Input: part model. Units: mm. Frame: model coordinates. A direction names the side the tool comes from. Give positions to 0.01 mm unless a question says otherwise; leave off trailing zeros. Loops run counter-clockwise (first coordinate to the right, second up) from the corner with the lowest first, then second, coordinate; pieces in that order, holes last. Notation, with made-up numbers: (-21.75, 16) -> (-7.75, 16) arc R29 cw to (-7.75, 51) -> close; hole circle Ø3 at (-13, -35). An arc over 180 degrees is marked (long way). One line per question, with ' | ' between items.
from build123d import *

# Parameters (mm, degrees)
EXTRUDE_THIN1_DEPTH             = 37.5
EXTRUDE_THIN1_DEPTH_BACK        = 37.5
CUT_EXTRUDE1_REACH              = 44.057
LPATTERN1_COUNT                 = 2
LPATTERN1_PITCH                 = 25
LPATTERN1_COL_COUNT             = 2
LPATTERN1_COL_PITCH             = 25
SCHNITT_LINEAR_START            = -11
SCHNITT_LINEAR_AUSTRAGEN1_DEPTH = 11


with BuildPart() as part:
    # Sketch1 → Extrude-Thin1 (new, two sides: drawn at the far end of the back side and taken through both)
    with BuildSketch(Plane(origin=(0, 0, 0), x_dir=(0, 0, -1), z_dir=(1, 0, 0)).offset(-EXTRUDE_THIN1_DEPTH_BACK)):
        with BuildLine():
            Line((-17.5, 6.5), (-15.5, 6.5))
            ThreePointArc((-15.5, 6.5), (-14.085786438, 5.914213562), (-13.5, 4.5))
            Line((-13.5, 4.5), (-13.5, 2))
            ThreePointArc((-13.5, 2), (-12.914213562, 0.585786438), (-11.5, 0))
            Line((-11.5, 0), (11.5, 0))
            ThreePointArc((11.5, 0), (12.914213562, 0.585786438), (13.5, 2))
            Line((13.5, 2), (13.5, 4.5))
            ThreePointArc((13.5, 4.5), (14.085786438, 5.914213562), (15.5, 6.5))
            Line((15.5, 6.5), (17.5, 6.5))
            Line((17.5, 6.5), (17.5, 7.5))
            Line((17.5, 7.5), (15.5, 7.5))
            ThreePointArc((15.5, 7.5), (13.378679656, 6.621320344), (12.5, 4.5))
            Line((12.5, 4.5), (12.5, 2))
            ThreePointArc((12.5, 2), (12.207106781, 1.292893219), (11.5, 1))
            Line((11.5, 1), (-11.5, 1))
            ThreePointArc((-11.5, 1), (-12.207106781, 1.292893219), (-12.5, 2))
            Line((-12.5, 2), (-12.5, 4.5))
            ThreePointArc((-12.5, 4.5), (-13.378679656, 6.621320344), (-15.5, 7.5))
            Line((-15.5, 7.5), (-17.5, 7.5))
            Line((-17.5, 7.5), (-17.5, 6.5))
        make_face()
    extrude(amount=EXTRUDE_THIN1_DEPTH + EXTRUDE_THIN1_DEPTH_BACK)

    # Sketch2 → Cut-Extrude1 (cut, up to next)
    with BuildSketch(Plane.XZ, mode=Mode.PRIVATE) as cut_extrude1_sk1:
        with BuildLine():
            Line((-5.875, 3.125), (5.875, 3.125))
            ThreePointArc((5.875, 3.125), (9, 0), (5.875, -3.125))
            Line((5.875, -3.125), (-5.875, -3.125))
            ThreePointArc((-5.875, -3.125), (-9, 0), (-5.875, 3.125))
        make_face()
    cut_extrude1_tool1 = extrude(cut_extrude1_sk1.sketch, amount=-CUT_EXTRUDE1_REACH, mode=Mode.PRIVATE) & part.part
    cut_extrude1 = cut_extrude1_tool1.solids().sort_by_distance((0, 0, 0))[0]
    add(cut_extrude1, mode=Mode.SUBTRACT)

    # LPattern1: Cut-Extrude1 ×2
    with Locations(*[(i * LPATTERN1_PITCH, 0, 0) for i in range(1, LPATTERN1_COUNT)]):
        add(cut_extrude1, mode=Mode.SUBTRACT)

    # LPattern1 col: Cut-Extrude1 ×2
    with Locations(*[(-i * LPATTERN1_COL_PITCH, 0, 0) for i in range(1, LPATTERN1_COL_COUNT)]):
        add(cut_extrude1, mode=Mode.SUBTRACT)

    # Skizze1 → Schnitt-Linear austragen1 (cut)
    with BuildSketch(Plane(origin=(37.5, 0, 0), x_dir=(0, 0, -1), z_dir=(1, 0, 0)).offset(SCHNITT_LINEAR_START)):
        with BuildLine():
            Line((-15.5, 7.5), (-17.5, 7.5))
            Line((-17.5, 7.5), (-17.5, 6.5))
            Line((-17.5, 6.5), (-15.5, 6.5))
            ThreePointArc((-15.5, 6.5), (-14.085786438, 5.914213562), (-13.5, 4.5))
            Line((-13.5, 4.5), (-13.5, 2))
            ThreePointArc((-13.5, 2), (-12.914213562, 0.585786438), (-11.5, 0))
            Line((-11.5, 0), (11.5, 0))
            ThreePointArc((11.5, 0), (12.914213562, 0.585786438), (13.5, 2))
            Line((13.5, 2), (13.5, 4.5))
            ThreePointArc((13.5, 4.5), (14.085786438, 5.914213562), (15.5, 6.5))
            Line((15.5, 6.5), (17.5, 6.5))
            Line((17.5, 6.5), (17.5, 7.5))
            Line((17.5, 7.5), (15.5, 7.5))
            ThreePointArc((15.5, 7.5), (13.378679656, 6.621320344), (12.5, 4.5))
            Line((12.5, 4.5), (12.5, 2))
            ThreePointArc((12.5, 2), (12.207106781, 1.292893219), (11.5, 1))
            Line((11.5, 1), (-11.5, 1))
            ThreePointArc((-11.5, 1), (-12.207106781, 1.292893219), (-12.5, 2))
            Line((-12.5, 2), (-12.5, 4.5))
            ThreePointArc((-12.5, 4.5), (-13.378679656, 6.621320344), (-15.5, 7.5))
        make_face()
    extrude(amount=SCHNITT_LINEAR_AUSTRAGEN1_DEPTH, mode=Mode.SUBTRACT)


solid = part.part
1. Section query B-B (z = 0). Output: boundary loops of the cut face in (x, y), then the cut area to 3 significant figures.
Determined:
outline: (-37.5, 0) -> (-34, 0) -> (-34, 1) -> (-37.5, 1) -> close; (-16, 0) -> (-9, 0) -> (-9, 1) -> (-16, 1) -> close; (9, 0) -> (16, 0) -> (16, 1) -> (9, 1) -> close | area: 17.5 mm2
2. Ray query, line 1 along Z through (x, y) = (20.5, 4.25); line 2 along Y through (x, z) = (22, -10.5); line 3 along Z through (x, y) = (-35, 7.25). Return the intervals inside material, ascending. Write a range as from..to.
Determined:
line 1: z = -13.5..-12.5, 12.5..13.5 | line 2: y = 0..1 | line 3: z = -17.5..-14.3, 14.3..17.5
3. Section query A-A (y = 3.5). Output: boundary loops of the cut face in (x, z).
Determined:
outline: (-37.5, -13.5) -> (26.5, -13.5) -> (26.5, -12.5) -> (-37.5, -12.5) -> close; (-37.5, 12.5) -> (26.5, 12.5) -> (26.5, 13.5) -> (-37.5, 13.5) -> close
4. Pull-direction query (Z, two-part tool) for faces 1 (the flat face through (-6, 3, -13.5)), 2 (the flat face through (-6, 6.5, -16)), 3 (the cylindrical face through (-16, 0.5, 0.1)); classes: pulls with the +Z half, pulls with the -Z half, needs draft (parallel to the pull), parting line crosses it, or undercut.
Determined:
face 1: pulls with the -Z half | face 2: needs draft | face 3: undercut
5. Section query C-C (x = -33). Output: boundary loops of the cut face in (y, z), then the cut area to 3 significant figures.
Determined:
outline: (0, -11.5) arc R2 ccw to (2, -13.5) -> (4.5, -13.5) arc R2 cw to (6.5, -15.5) -> (6.5, -17.5) -> (7.5, -17.5) -> (7.5, -15.5) arc R3 ccw to (4.5, -12.5) -> (2, -12.5) arc R1 cw to (1, -11.5) -> (1, -2.29) -> (0, -2.29) -> close; (0, 2.29) -> (1, 2.29) -> (1, 11.5) arc R1 cw to (2, 12.5) -> (4.5, 12.5) arc R3 ccw to (7.5, 15.5) -> (7.5, 17.5) -> (6.5, 17.5) -> (6.5, 15.5) arc R2 cw to (4.5, 13.5) -> (2, 13.5) arc R2 ccw to (0, 11.5) -> close | area: 40.0 mm2
6. Section query D-D (x = 13). Output: boundary loops of the cut face in (y, z).
Determined:
outline: (0, -11.5) arc R2 ccw to (2, -13.5) -> (4.5, -13.5) arc R2 cw to (6.5, -15.5) -> (6.5, -17.5) -> (7.5, -17.5) -> (7.5, -15.5) arc R3 ccw to (4.5, -12.5) -> (2, -12.5) arc R1 cw to (1, -11.5) -> (1, 11.5) arc R1 cw to (2, 12.5) -> (4.5, 12.5) arc R3 ccw to (7.5, 15.5) -> (7.5, 17.5) -> (6.5, 17.5) -> (6.5, 15.5) arc R2 cw to (4.5, 13.5) -> (2, 13.5) arc R2 ccw to (0, 11.5) -> close
7. Reachability of faces 4 (the flat face through (-6, 3, -12.5)), 5 (the flat face through (-6, 6.5, 17)), 6 (the cylindrical face through (-9, 0.5, -0.1)) from +Z, -Z, +X, -X, +Y, -Y: full face, straight path, thin tool, end or side. Return the list, or none.
Determined:
face 4: +X, -X, +Y | face 5: +Z, +X, -X, -Y | face 6: +Y, -Y
8. Pin query (flat end, axial travel): P1, Ø3, axis at x = -7, y = 3.5, coming from the +Z side; P2, Ø0.8, axis at x = -3, y = 3.5, coming from the -Z side; P3, Ø0.5, axis at x = 22.5, y = 0.5, coming from the -Z side; P4, Ø8, axis at x = -6, z = -12, coming from the -Y side. Return the tip coordinate at first contact, or that it passes through.
Determined:
P1: stops at z = 13.56 | P2: stops at z = -13.5 | P3: stops at z = -13.06 | P4: stops at y = 0
